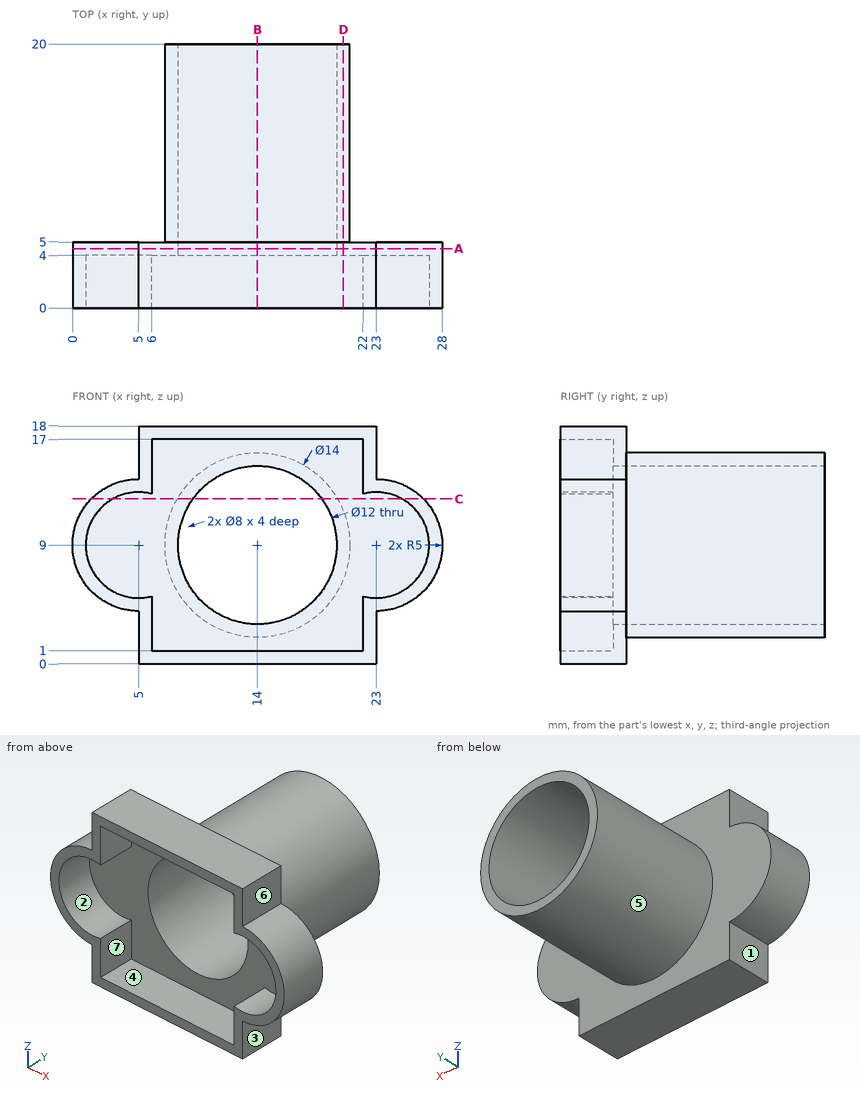
Geometry check sheet. Reference: drawing and pictorial views, mm from the part's lowest x, y, z. A direction names the side the tool comes from. Give positions to 0.01 mm unless a question says otherwise; leave off trailing zeros. Write each loop counter-clockwise with the first axis right and the second up, starting at its lowest first coordinate (ties: lowest second). Pieces come first, ordered by that corner, then holes.
Item 1: Cross-section at A-A (y = 4.5). Enter the section's corners in (x, z).
Item 2: Cross-section at B-B (x = 14). Enter the section's corners in (y, z).
Item 3: Draft check along X on the marked faces 1, 2, 3 and 4. Enter one of: released by +X, released by -X, zero draft, split by the parting line, or undercut.
Item 4: Access from +Z, -Z, +X, -X, +Y, -Y to the whole of each face (thin tool, end or side, straight path). Record for the marked faces 5, 6 and 7.
Item 5: Scan lines: L1, parallel to Z at x = 14, y = 11.5; L2, parallel to X at y = 8, z = 9; L3, parallel to X at y = 3.1, z = 9. Record each from-to range of solid material in increasing order.
Item 6: Gauge pin test, flat ends, axial feed: pin 1 (8 mm diameter, centred on x = 12, z = 8, fed in from -Y); pin 2 (1.2 mm diameter, centred on y = 3, z = 15.5, fed in from -X); pin 3 (7 mm diameter, centred on x = 14, z = 9, fed in from +Y); pin 4 (2 mm diameter, centred on x = 14.5, y = 17.5, fed in from -Z). Record the tip position at first contact, or that the pin passes through.
Item 7: Cross-section at C-C (z = 12.5). Enter the section's corners in (x, y).
Item 8: Cross-section at D-D (x = 20.5). Enter the section's corners in (y, z).
Report:
1. outline: (5, 0) - (23, 0) - (23, 4) arc R5 ccw to (23, 14) - (23, 18) - (5, 18) - (5, 14) arc R5 ccw to (5, 4) - close; hole circle Ø12 at (14, 9)
2. outline: (0, 0) - (5, 0) - (5, 2) - (20, 2) - (20, 3) - (4, 3) - (4, 1) - (0, 1) - close; (0, 17) - (4, 17) - (4, 15) - (20, 15) - (20, 16) - (5, 16) - (5, 18) - (0, 18) - close
3. face 1: released by -X
3. face 2: undercut
3. face 3: released by +X
3. face 4: undercut
4. face 5: +Y
4. face 6: +Z, +X, +Y, -Y
4. face 7: -Y
5. L1: z = 2 to 3, 15 to 16
5. L2: x = 7 to 8, 20 to 21
5. L3: x = 0 to 1, 27 to 28
6. pin 1: stops at y = 4
6. pin 2: stops at x = 5
6. pin 3: passes through
6. pin 4: stops at z = 2
7. outline: (1.43, 0) - (3.06, 0) - (3.06, 4) - (9.13, 4) - (9.13, 20) - (7.94, 20) - (7.94, 5) - (1.43, 5) - close; (18.87, 4) - (24.94, 4) - (24.94, 0) - (26.57, 0) - (26.57, 5) - (20.06, 5) - (20.06, 20) - (18.87, 20) - close
8. outline: (0, 0) - (5, 0) - (5, 6.4) - (20, 6.4) - (20, 11.6) - (5, 11.6) - (5, 18) - (0, 18) - (0, 17) - (4, 17) - (4, 1) - (0, 1) - close
